Verification items for the finished model (mm, model axes). A direction names the side the tool comes from. Give positions to 0.01 mm unless a question says otherwise; leave off trailing zeros. Write each loop counter-clockwise with the first axis right and the second up, starting at its lowest first coordinate (ties: lowest second). Pieces come first, ordered by that corner, then holes. Notation, with made-up numbers: (-11, -19) - (-4, -19) arc R6 cw to (-4, -10) - close; hole circle Ø2 at (-21.5, 89.25). An arc over 180 degrees is marked (long way). Answer as a JSON object with one key per item and string values. Group by question number.
Item 1: Draft check along Z on faces 1 (the face through (3, -131, 6.691)), 2 (the face through (3, 37.957, -7)), 3 (the face through (3, -52, -138.197)). Enter one of: +Z half, -Z half, draft (parallel to the pull), parting line (faces both ways), or undercut.
Item 2: Go/stop test with flat-tipped pins: pin 1 (0.7 mm diameter, centred on x = 2.5, z = -108, fed in from +Y); pin 2 (1.5 mm diameter, centred on x = 2.5, y = 41, fed in from +Z). Record where each tip stops, or that it passes through.
Item 3: Tool access check on faces 4 (the face through (3, 36, -109.192)), 5 (the face through (3, 37.957, -125)), 6 (the face through (3, -131, -109.192)). Record the directions out of +Z, -Z, +X, -X, +Y, -Y that give a thin tool (end or side, any length) a straight path to the whole face; none if there is none.
Item 4: Scan lines: line 1 along Z through (x, y) = (2.1, 34); line 2 along Y through (x, z) = (1, 21); line 3 along Y through (x, z) = (3.85, 9). Record each from-to range of solid material in increasing order. Write a range as [from, to].
Item 5: Sectioned sample at A-A, the plane z = -17.5. Record the boundary of the cut face in (x, y).
```python
from build123d import *

# Parameters (mm, degrees)
SKETCH1_W            = 173.89
SKETCH1_H            = 177.8
MAIN_DEPTH           = 5.13
T_SLOT_DEPTH         = 5.13
LPATTERN2_COUNT      = 2
LPATTERN2_PITCH      = 118.88
MIRROR1_COPY_1_DEPTH = 5.13
SKETCH6_W            = 5.13
SKETCH6_H            = 58.88
TOOTH_DEPTH          = 5.13


with BuildPart() as part:
    # Sketch1 → Main (new body)
    with BuildSketch(Plane(origin=(0, 0, 0), x_dir=(0, 0, -1), z_dir=(1, 0, 0))):
        with Locations((51.252197546, -50.943101868)):
            Rectangle(SKETCH1_W, SKETCH1_H)
    extrude(amount=MAIN_DEPTH)

    # Sketch2 → t-slot (cut)
    with BuildSketch(Plane(origin=(5.13, 0, 0), x_dir=(0, 0, -1), z_dir=(1, 0, 0))):
        Polygon((-9.687802454, 37.956898132), (-6.690802454, 37.956898132), (-6.690802454, 33.961898132), (-5.331802454, 33.961898132), (-5.331802454, 31.794898132), (-6.690802454, 31.794898132), (-6.690802454, 25.587898132), (-9.687802454, 25.587898132), (-9.687802454, 31.794898132), (-11.046802454, 31.794898132), (-11.046802454, 33.961898132), (-9.687802454, 33.961898132), align=None)
    t_slot = extrude(amount=-T_SLOT_DEPTH, mode=Mode.SUBTRACT)

    # LPattern2: t-slot ×2
    with Locations(*[(0, 0, -i * LPATTERN2_PITCH) for i in range(1, LPATTERN2_COUNT)]):
        add(t_slot, mode=Mode.SUBTRACT)

    # Mirror1: t-slot across plane
    add(t_slot.mirror(Plane(origin=(0, -50.943101868, 0), x_dir=(0, 0, 1), z_dir=(0, -1, 0))), mode=Mode.SUBTRACT)

    # Mirror1 copy 1 sketch → Mirror1 copy 1 (cut)
    with BuildSketch(Plane(origin=(5.13, -101.886203737, -118.88), x_dir=(0, 0, -1), z_dir=(1, 0, 0))):
        Polygon((-9.687802454, -37.956898132), (-6.690802454, -37.956898132), (-6.690802454, -33.961898132), (-5.331802454, -33.961898132), (-5.331802454, -31.794898132), (-6.690802454, -31.794898132), (-6.690802454, -25.587898132), (-9.687802454, -25.587898132), (-9.687802454, -31.794898132), (-11.046802454, -31.794898132), (-11.046802454, -33.961898132), (-9.687802454, -33.961898132), align=None)
    extrude(amount=-MIRROR1_COPY_1_DEPTH, mode=Mode.SUBTRACT)

    # Sketch6 → Tooth (add)
    with BuildSketch(Plane(origin=(0, 37.956898132, 0), x_dir=(1, 0, 0), z_dir=(0, 1, 0))):
        with Locations((2.565, 51.252197546)):
            Rectangle(SKETCH6_W, SKETCH6_H)
    extrude(amount=TOOTH_DEPTH)


solid = part.part
```
Geometry check:
{
 "1": {"face 1": "undercut", "face 2": "draft", "face 3": "-Z half"},
 "2": {"pin 1": "y = 37.96", "pin 2": "z = -21.81"},
 "3": {"face 4": "+X, -X, +Y", "face 5": "-Z, +X, -X, +Y", "face 6": "+X, -X, -Y"},
 "4": {"line 1": "[-138.2, -112.19], [-109.19, 6.69], [9.69, 35.69]", "line 2": "[-139.84, 37.96]", "line 3": "[-127.47, 25.59]"},
 "5": {"outline": "(0, -139.84) - (5.13, -139.84) - (5.13, 37.96) - (0, 37.96) - close"}
}
